from build123d import *

# Parameters (mm, degrees)
F0_R      = 19
F1_DEPTH  = 17
F2_R      = 17
F2_R_2    = 10.5
F3_DEPTH  = 15
F4_R      = 3
F5_DEPTH  = 10
F6_R      = 10
F7_DEPTH  = 12
F8_R      = 2
F9_DEPTH  = 25
F10_DEPTH = 4
F8_R_2    = 4
F11_DEPTH = 2
F12_R     = 11
F13_DEPTH = 0.25
F14_R     = 2
F15_DEPTH = 4


with BuildPart() as f1:
    # F0 (on Top) → F1 (new body)
    with BuildSketch(Plane.XY):
        with Locations((19, 19)):
            Circle(F0_R)
    extrude(amount=F1_DEPTH)

    # F2 (on Top) → F3 (cut)
    with BuildSketch(Plane.XY):
        with Locations((19, 19)):
            Circle(F2_R)
        with Locations((19, 19)):
            Circle(F2_R_2, mode=Mode.SUBTRACT)
    extrude(amount=F3_DEPTH, mode=Mode.SUBTRACT)

    # F4 (on face) → F5 (join)
    with BuildSketch(Plane.XY):
        with Locations((19.039284, 18.877556)):
            Circle(F4_R)
    extrude(amount=-F5_DEPTH)

    # F6 (on face) → F7 (cut)
    with BuildSketch(Plane.XY.offset(17)):
        with Locations((19, 19)):
            Circle(F6_R)
    extrude(amount=-F7_DEPTH, mode=Mode.SUBTRACT)

    # F8 (on face) → F9 (cut)
    with BuildSketch(Plane.XY.offset(5)):
        with Locations((19, 26)):
            Circle(F8_R)
        with Locations((23.962697, 23.936764)):
            Circle(F8_R)
        with Locations((26, 19)):
            Circle(F8_R)
        with Locations((24.39163, 14.535661)):
            Circle(F8_R)
        with Locations((19, 12)):
            Circle(F8_R)
        with Locations((13.836625, 14.273526)):
            Circle(F8_R)
        with Locations((12, 19)):
            Circle(F8_R)
        with Locations((14.063236, 23.962697)):
            Circle(F8_R)
    extrude(amount=-F9_DEPTH, mode=Mode.SUBTRACT)

    # F8 (on face) → F10 (join)
    with BuildSketch(Plane.XY.offset(5)):
        with Locations((19, 19)):
            Circle(F8_R)
    extrude(amount=F10_DEPTH)

    # F8 (on face) → F11 (join)
    with BuildSketch(Plane.XY.offset(5)):
        with Locations((19, 19)):
            Circle(F8_R_2)
        with Locations((19, 19)):
            Circle(F8_R, mode=Mode.SUBTRACT)
    extrude(amount=F11_DEPTH)

    # F12 (on face) → F13 (cut)
    with BuildSketch(Plane.XY.offset(17)):
        with Locations((19.02286, 19.252149)):
            Circle(F12_R)
    extrude(amount=-F13_DEPTH, mode=Mode.SUBTRACT)

    # F14 (on face) → F15 (cut)
    with BuildSketch(Plane(origin=(0, 0, -10), x_dir=(1, 0, 0), z_dir=(0, 0, -1))):
        with Locations((19.039284, -18.877556)):
            Circle(F14_R)
    extrude(amount=-F15_DEPTH, mode=Mode.SUBTRACT)


solid = f1.part
Part model, mm, in its own coordinate system. A direction names the side the tool comes from. Give positions to 0.01 mm unless a question says otherwise; leave off trailing zeros. Loops run counter-clockwise (first coordinate to the right, second up) from the corner with the lowest first, then second, coordinate; pieces in that order, holes last. Notation, with made-up numbers: (75.5, 69) -> (128.5, 69) arc R21 ccw to (128.5, 107) -> close; hole circle Ø7 at (-2, 32.5). An arc over 180 degrees is marked (long way). Write each question's results on one line, items separated by ' | '. Start each with the question number.
Q1. Wall check: L1, parallel to X at y = 15.5, z = 3.5; L2, parallel to Y at x = 11, z = 13; L3, parallel to X at y = 15, z = 10. Give the ranges that are in metal, low to high.
Q2. Band-saw the part on A-A on z = 8. List the corners of the cut face in (x, y).
Q3. Band-saw the part on B-B on z = 3.75. Count the separate pieces of the cut face and the enclosed holes in it, plus the area to 3 significant figures.
Q4. Which spindle directions (+Z, -Z, +X, -X, +Y, -Y) get a long thin tool onto all of the face, cutting with end or side? Do faces 4 (the face through (25.31, 12.76, 2.54)), 5 (the face through (17, 29, 16.75)), 6 (the face through (19, 19, -6)). Say none if no direction does.
Q5. Pin check, flat tips, straight feed: P1, Ø10, axis at x = 27, y = 22, coming from the -Z side; P2, Ø1, axis at x = 14, z = 10, coming from the +Y side; P3, Ø3, axis at x = 19, y = 19.5, coming from the +Z side. Stop position of each tip, or through.
Q6. Pull direction X, two halves, no side cores. Call faces 1 (the face through (17, 18, 7)), 2 (the face through (29.214, 35.021, 8.381)), 3 (the face through (5, 9, 0)): +X half, -X half, draft (parallel to the pull), parting line (faces both ways), or undercut.
Results are:
1) L1: x = 0.33 to 2.36, 9.1 to 12.26, 15.42 to 22.64, 26.14 to 28.9, 35.64 to 37.67 | L2: y = 1.77 to 4, 12.2 to 13, 25 to 25.8, 34 to 36.23 | L3: x = 0.43 to 2.48, 9.29 to 9.83, 28.17 to 28.71, 35.52 to 37.57
2) outline: circle Ø38 at (19, 19); circle Ø21 at (19, 19); circle Ø4 at (19, 19); hole circle Ø34 at (19, 19); hole circle Ø20 at (19, 19)
3) separate pieces: 2 | enclosed holes: 9 | area: 472 mm²
4) face 4: +Z, -Z | face 5: +Z | face 6: -Z
5) P1: stops at z = 0 | P2: stops at y = 37.46 | P3: stops at z = 9
6) face 1: undercut | face 2: parting line | face 3: draft
